The model under review builds one solid part; all positions refer to its coordinate system, in mm. A direction names the side the tool comes from. Coordinates: 2 decimals unless noted, no trailing zeros. Write each loop counter-clockwise with the first axis right and the second up, starting at its lowest first coordinate (ties: lowest second). Pieces come first, ordered by that corner, then holes. Notation, with made-up numbers: (35, -2.75) -> (51, -2.75) arc R24 cw to (51, 9.25) -> close; hole circle Ø2 at (32.5, 47). An arc over 180 degrees is marked (long way). Write each question's results on one line, items separated by ' | '.
```python
from build123d import *

# Parameters (mm, degrees)
BOSS_EXTRUDE1_DEPTH            = 3.175
F_3_16_0_1875_DIAMETER_HOLE1_D = 4.7625
SKETCH6_W                      = 3.175
SKETCH6_H                      = 12.7
BOSS_EXTRUDE2_DEPTH            = 12.7
F_9_0_196_DIAMETER_HOLE1_D     = 4.9784
SKETCH9_W                      = 6.35
SKETCH9_H                      = 2.35
SKETCH9_H_2                    = 3.175
SKETCH9_H_3                    = 1.95
BOSS_EXTRUDE3_DEPTH            = 12.7
CUT_EXTRUDE1_DEPTH             = 67.530730681
SKETCH11_W                     = 3.175
SKETCH11_H                     = 6.35
BOSS_EXTRUDE4_DEPTH            = 12.7


with BuildPart() as part:
    # Sketch1 → Boss-Extrude1 (new body)
    with BuildSketch(Plane(origin=(0, 0, 0), x_dir=(1, 0, 0), z_dir=(0, 1, 0))):
        Polygon((0.4, -0.4), (0.4, 42), (6.75, 42), (6.75, -0.4), (4.4, -25.8), (-46.4, -25.8), (-48.75, -0.4), (-48.75, 42), (-42.4, 42), (-42.4, -0.4), align=None)
    extrude(amount=BOSS_EXTRUDE1_DEPTH)

    # 3/16 (0.1875) Diameter Hole1 (through all)
    with Locations(Plane(origin=(0, 3.175, 0), x_dir=(1, 0, 0), z_dir=(0, 1, 0))):
        with Locations((-33.7, -13.178131577), (-8.3, -13.178131577)):
            Hole(F_3_16_0_1875_DIAMETER_HOLE1_D / 2)

    # Sketch6 → Boss-Extrude2 (add)
    with BuildSketch(Plane(origin=(0, 3.175, 0), x_dir=(1, 0, 0), z_dir=(0, 1, 0))):
        with Locations((-43.9875, 8.3)):
            Rectangle(SKETCH6_W, SKETCH6_H)
        with Locations((-43.9875, 33.7)):
            Rectangle(SKETCH6_W, SKETCH6_H)
        with Locations((1.9875, 8.3)):
            Rectangle(SKETCH6_W, SKETCH6_H)
        with Locations((1.9875, 33.7)):
            Rectangle(SKETCH6_W, SKETCH6_H)
    extrude(amount=BOSS_EXTRUDE2_DEPTH)

    # #9 (0.196) Diameter Hole1 (through all)
    with Locations(Plane.ZY.offset(45.575)):
        with Locations((-8.3, 10.1854), (-33.7, 10.1854)):
            Hole(F_9_0_196_DIAMETER_HOLE1_D / 2)

    # Sketch9 → Boss-Extrude3 (add)
    with BuildSketch(Plane(origin=(0, 3.175, 0), x_dir=(1, 0, 0), z_dir=(0, 1, 0))):
        with Locations((-45.575, 0.775)):
            Rectangle(SKETCH9_W, SKETCH9_H)
        with Locations((3.575, 0.775)):
            Rectangle(SKETCH9_W, SKETCH9_H)
        with Locations((3.575, 16.2375)):
            Rectangle(SKETCH9_W, SKETCH9_H_2)
        with Locations((-45.575, 16.2375)):
            Rectangle(SKETCH9_W, SKETCH9_H_2)
        with Locations((3.575, 25.7625)):
            Rectangle(SKETCH9_W, SKETCH9_H_2)
        with Locations((3.575, 41.025)):
            Rectangle(SKETCH9_W, SKETCH9_H_3)
        with Locations((-45.575, 41.025)):
            Rectangle(SKETCH9_W, SKETCH9_H_3)
        with Locations((-45.575, 25.7625)):
            Rectangle(SKETCH9_W, SKETCH9_H_2)
    extrude(amount=BOSS_EXTRUDE3_DEPTH)

    # Sketch10 → Cut-Extrude1 (cut, through all)
    with BuildSketch(Plane.XY.offset(0.4)):
        Polygon((-48.75, 3.175), (-45.575, 15.875), (-48.75, 15.875), align=None)
        Polygon((6.75, 3.175), (3.575, 15.875), (6.75, 15.875), align=None)
    extrude(amount=-CUT_EXTRUDE1_DEPTH, mode=Mode.SUBTRACT)

    # Sketch11 → Boss-Extrude4 (add)
    with BuildSketch(Plane(origin=(0, 3.175, 0), x_dir=(1, 0, 0), z_dir=(0, 1, 0))):
        with Locations((-43.9875, 21)):
            Rectangle(SKETCH11_W, SKETCH11_H)
        with Locations((1.9875, 21)):
            Rectangle(SKETCH11_W, SKETCH11_H)
    extrude(amount=BOSS_EXTRUDE4_DEPTH)


solid = part.part
```
Q1. Add section C-C (z = -0.5). Write out the cut boundary in (x, y) (3 decimals), plus the area to 3 significant figures.
Solution:
outline: (-48.75, 0) -> (-42.4, 0) -> (-42.4, 15.875) -> (-45.575, 15.875) -> (-48.75, 3.175) -> close; (0.4, 0) -> (6.75, 0) -> (6.75, 3.175) -> (3.575, 15.875) -> (0.4, 15.875) -> close | area: 161 mm²
Q2. Machinability: for faces 4 (the flat face through (6.75, 2, -21)), 5 (the flat face through (-46, 7, -17.825)), 6 (the flat face through (3, 9, 0.4)), which of the approach directions +Z, -Z, +X, -X, +Y, -Y give a long, thin tool a straight path to every point of the face, cutting with its end or side? Answer none if there is none.
Solution:
face 4: +Z, -Z, +X, +Y, -Y | face 5: -X, +Y | face 6: +Z, +X, -X, +Y
Q3. Draft analysis for pull direction Z (two halves, no side actions). For faces 1 (the flat face through (5, 8, -40.05)), 2 (the flat face through (-47.185, 9.436, -16.215)), 3 (the flat face through (5.59, 1.57, 12.92)), state which applies: pulls with the +Z half, pulls with the -Z half, needs draft (parallel to the pull), parting line crosses it, or undercut.
Solution:
face 1: undercut | face 2: needs draft | face 3: pulls with the +Z half
Q4. Add section A-A (z = -33.7). Write out the cut boundary in (x, y) (3 decimals), plus the area to 3 significant figures.
Solution:
outline: (-48.75, 0) -> (-42.4, 0) -> (-42.4, 7.696) -> (-45.575, 7.696) -> (-45.575, 3.175) -> (-48.75, 3.175) -> close; (-45.575, 12.675) -> (-42.4, 12.675) -> (-42.4, 15.875) -> (-45.575, 15.875) -> close; (0.4, 0) -> (6.75, 0) -> (6.75, 3.175) -> (3.575, 3.175) -> (3.575, 7.696) -> (0.4, 7.696) -> close; (0.4, 12.675) -> (3.575, 12.675) -> (3.575, 15.875) -> (0.4, 15.875) -> close | area: 89.4 mm²
Q5. For line 1 (X direction, y = 8.75, z = -29) (3 decimals); line 2 (Y direction, x = 1.15, z = -33.7) (3 decimals); line 3 (Z direction, x = -33.7, y = 1.9), list the stretches that pass through material, from the lowest coordinate up. Write a range as from..to.
Solution:
line 1: -45.575..-42.4, 0.4..3.575 | line 2: 0..7.696, 12.675..15.875 | line 3: 0.4..10.8, 15.56..25.8
Q6. Add section B-B (x = -8.3). Write out the cut boundary in (y, z) (3 decimals), plus the area to 3 significant figures.
Solution:
outline: (0, 0.4) -> (3.175, 0.4) -> (3.175, 10.797) -> (0, 10.797) -> close; (0, 15.559) -> (3.175, 15.559) -> (3.175, 25.8) -> (0, 25.8) -> close | area: 65.5 mm²
Q7. Clearance check with flat-ended pins moving along their axes: P1, Ø5.5, axis at y = 10.19, z = -33.7, coming from the +X side (3 decimals); P2, Ø1.6, axis at x = 5.5, z = -6, coming from the +Y side (3 decimals); P3, Ø7, axis at x = -46.5, y = 8, coming from the +Z side. State where each tip first meets the part, or that it passes through.
Solution:
P1: x = 3.575 | P2: y = 3.175 | P3: z = 0.4
Q8. Add section D-D (x = -34.5). Write out the cut boundary in (y, z) (3 decimals).
Solution:
outline: (0, 0.4) -> (3.175, 0.4) -> (3.175, 10.935) -> (0, 10.935) -> close; (0, 15.421) -> (3.175, 15.421) -> (3.175, 25.8) -> (0, 25.8) -> close
